```python
from build123d import *

# Parameters (mm, degrees)
SKETCH_W        = 15.8
SKETCH_H        = 9.6
PAD_DEPTH       = 10
SKETCH002_W     = 15
SKETCH002_H     = 12
PAD001_DEPTH    = 1
SKETCH003_W     = 3
SKETCH003_H     = 6
POCKET_DEPTH    = 9
SKETCH004_W     = 3
SKETCH004_H     = 6
POCKET001_DEPTH = 9
POCKET002_DEPTH = 11.001
POCKET003_DEPTH = 11.001
POCKET004_DEPTH = 11.001
POCKET005_DEPTH = 11.001


with BuildPart() as part:
    # Sketch → Pad (new body)
    with BuildSketch(Plane.XY):
        Rectangle(SKETCH_W, SKETCH_H)
    extrude(amount=PAD_DEPTH)

    # Sketch002 → Pad001 (join)
    with BuildSketch(Plane(origin=(0, 0, 0), x_dir=(1, 0, 0), z_dir=(0, 0, -1))):
        Rectangle(SKETCH002_W, SKETCH002_H)
    extrude(amount=PAD001_DEPTH)

    # Sketch003 → Pocket (cut)
    with BuildSketch(Plane(origin=(0, 0, -2), x_dir=(1, 0, 0), z_dir=(0, 0, -1))):
        with Locations((-2.5, 0)):
            Rectangle(SKETCH003_W, SKETCH003_H)
    extrude(amount=-POCKET_DEPTH, mode=Mode.SUBTRACT)

    # Sketch004 → Pocket001 (cut)
    with BuildSketch(Plane(origin=(0, 0, -2), x_dir=(1, 0, 0), z_dir=(0, 0, -1))):
        with Locations((2.5, 0)):
            Rectangle(SKETCH004_W, SKETCH004_H)
    extrude(amount=-POCKET001_DEPTH, mode=Mode.SUBTRACT)

    # Sketch001 → Pocket002 (cut, through all)
    with BuildSketch(Plane.XY.offset(10)):
        Polygon((3.32, -0.5), (3.32, -2.95), (0.5, -2.95), (0.5, -2.45), (2.76, -2.45), (2.76, -0.5), align=None)
    extrude(amount=-POCKET002_DEPTH, mode=Mode.SUBTRACT)

    # Sketch005 → Pocket003 (cut, through all)
    with BuildSketch(Plane.XY.offset(10)):
        Polygon((-3.32, -0.5), (-3.32, -2.95), (-0.5, -2.95), (-0.5, -2.45), (-2.76, -2.45), (-2.76, -0.5), align=None)
    extrude(amount=-POCKET003_DEPTH, mode=Mode.SUBTRACT)

    # Sketch007 → Pocket004 (cut, through all)
    with BuildSketch(Plane.XY.offset(10)):
        Polygon((-2.76, 0.5), (-3.32, 0.5), (-3.32, 2.95), (-0.5, 2.95), (-0.5, 2.39), (-2.76, 2.39), align=None)
    extrude(amount=-POCKET004_DEPTH, mode=Mode.SUBTRACT)

    # Sketch006 → Pocket005 (cut, through all)
    with BuildSketch(Plane.XY.offset(10)):
        Polygon((0.5, 2.95), (3.32, 2.95), (3.32, 0.5), (2.76, 0.5), (2.76, 2.45), (0.5, 2.45), align=None)
    extrude(amount=-POCKET005_DEPTH, mode=Mode.SUBTRACT)


solid = part.part
```
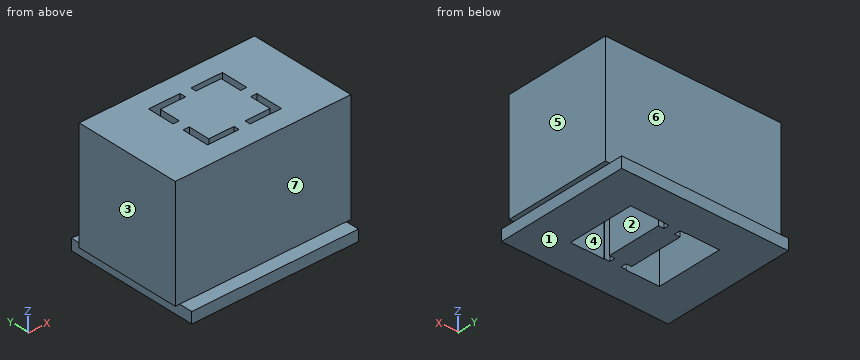
Input: part model. Units: mm. Frame: model coordinates. Face numbers are marked on the shaded views. A direction names the side the tool comes from. Coordinates: 2 decimals unless noted, no trailing zeros. Write each loop counter-clockwise with the first axis right and the second up, starting at its lowest first coordinate (ties: lowest second). Pieces come first, ordered by that corner, then holes.
1) Pin query (flat end, axial travel): pin 1 Ø3 at (x, z) = (-1, 3) entering from +Y; pin 2 Ø5 at (x, z) = (5, 6.5) entering from -Y. Return the tip coordinate at first contact, or that it passes through.
2) Section A-A on x = -2.5. Output: boundary loops of the cut face in (y, z).
3) Material intervals for line 1 along X through (y, z) = (2.25, 2); line 2 along X through (y, z) = (-0.25, -0.25); line 3 along Y through (x, z) = (2.5, 7.75), sorted ascending.
4) Section C-C on z = 1.75. Output: boundary loops of the cut face in (x, y).
5) Mould query, pull axis X, two halves, no side actions, for the marked faces 1, 2 and 3. Classes: pulls with the +X half, pulls with the -X half, needs draft (parallel to the pull), parting line crosses it, or undercut.
6) Section D-D on z = 7.5. Output: boundary loops of the cut face in (x, y).
7) Set-up query: the marked faces 4, 5, 6 and 7. Return all of +Z, -Z, +X, -X, +Y, -Y with unobstructed straight access to the full face (end or side cutting, diameter ignored); none if empty.
8) Section B-B on y = -2.25. Output: boundary loops of the cut face in (x, z), and give its area (3 significant figures).
Check result:
1. pin 1: stops at y = 4.8
1. pin 2: stops at y = -4.8
2. outline: (-6, -1) - (-3, -1) - (-3, 7) - (-2.95, 7) - (-2.95, 10) - (-4.8, 10) - (-4.8, 0) - (-6, 0) - close; (-2.45, 7) - (2.39, 7) - (2.39, 10) - (-2.45, 10) - close; (2.95, 7) - (3, 7) - (3, -1) - (6, -1) - (6, 0) - (4.8, 0) - (4.8, 10) - (2.95, 10) - close
3. line 1: x = -7.9 to -4, -1 to 1, 4 to 7.9
3. line 2: x = -7.5 to -4, -1 to 1, 4 to 7.5
3. line 3: y = -4.8 to -2.95, -2.45 to 2.45, 2.95 to 4.8
4. outline: (-7.9, -4.8) - (7.9, -4.8) - (7.9, 4.8) - (-7.9, 4.8) - close; hole (-4, -3) - (-1, -3) - (-1, -2.95) - (-0.5, -2.95) - (-0.5, -2.45) - (-1, -2.45) - (-1, 2.39) - (-0.5, 2.39) - (-0.5, 2.95) - (-1, 2.95) - (-1, 3) - (-4, 3) - close; hole (0.5, -2.95) - (1, -2.95) - (1, -3) - (4, -3) - (4, 3) - (1, 3) - (1, 2.95) - (0.5, 2.95) - (0.5, 2.45) - (1, 2.45) - (1, -2.45) - (0.5, -2.45) - close
5. face 1: needs draft
5. face 2: undercut
5. face 3: pulls with the -X half
6. outline: (-7.9, -4.8) - (7.9, -4.8) - (7.9, 4.8) - (-7.9, 4.8) - close; hole (-3.32, -2.95) - (-0.5, -2.95) - (-0.5, -2.45) - (-2.76, -2.45) - (-2.76, -0.5) - (-3.32, -0.5) - close; hole (-3.32, 0.5) - (-2.76, 0.5) - (-2.76, 2.39) - (-0.5, 2.39) - (-0.5, 2.95) - (-3.32, 2.95) - close; hole (0.5, -2.95) - (3.32, -2.95) - (3.32, -0.5) - (2.76, -0.5) - (2.76, -2.45) - (0.5, -2.45) - close; hole (0.5, 2.45) - (2.76, 2.45) - (2.76, 0.5) - (3.32, 0.5) - (3.32, 2.95) - (0.5, 2.95) - close
7. face 4: -Z
7. face 5: +Z, -Z, +X, +Y, -Y
7. face 6: +Z, +X, -X, +Y
7. face 7: +Z, +X, -X, -Y
8. outline: (-7.9, 0) - (-7.5, 0) - (-7.5, -1) - (-4, -1) - (-4, 7) - (-3.32, 7) - (-3.32, 10) - (-7.9, 10) - close; (-2.76, 7) - (-1, 7) - (-1, -1) - (1, -1) - (1, 7) - (2.76, 7) - (2.76, 10) - (-2.76, 10) - close; (3.32, 7) - (4, 7) - (4, -1) - (7.5, -1) - (7.5, 0) - (7.9, 0) - (7.9, 10) - (3.32, 10) - close
8. area: 122 mm2
